Build history of the part. All positions in model axes, mm. Give positions to 0.01 mm unless a question says otherwise; leave off trailing zeros. Loops run counter-clockwise (first coordinate to the right, second up) from the corner with the lowest first, then second, coordinate; pieces in that order, holes last. Notation, with made-up numbers: (74.5, 0.25) -> (111.5, 0.25) arc R27 cw to (111.5, 35.25) -> close; hole circle Ø3 at (-29, 56.25). An arc over 180 degrees is marked (long way). Answer in a Markdown table with one row per item. Add a question column.
from build123d import *

# Parameters (mm, degrees)
ESQUISSE1_R                  = 3.5
ESQUISSE1_R_2                = 3
BOSS_EXTRU_1_DEPTH           = 314
ESQUISSE2_R                  = 1
ENL_V_MAT_EXTRU_1_DEPTH      = 10
ENL_V_MAT_EXTRU_1_DEPTH_BACK = 10


with BuildPart() as part:
    # Esquisse1 → Boss.-Extru.1 (new body)
    with BuildSketch(Plane.XY):
        Circle(ESQUISSE1_R)
        Circle(ESQUISSE1_R_2, mode=Mode.SUBTRACT)
    extrude(amount=BOSS_EXTRU_1_DEPTH)

    # Esquisse2 → Enl_v. mat.-Extru.1 (cut, two sides)
    with BuildSketch(Plane(origin=(0, 0, 0), x_dir=(1, 0, 0), z_dir=(0, 1, 0))) as enl_v_mat_extru_1_sk:
        with Locations((0, -309)):
            Circle(ESQUISSE2_R)
        with Locations((0, -5)):
            Circle(ESQUISSE2_R)
    extrude(amount=ENL_V_MAT_EXTRU_1_DEPTH, mode=Mode.SUBTRACT)
    extrude(enl_v_mat_extru_1_sk.sketch, amount=-ENL_V_MAT_EXTRU_1_DEPTH_BACK, mode=Mode.SUBTRACT)


solid = part.part
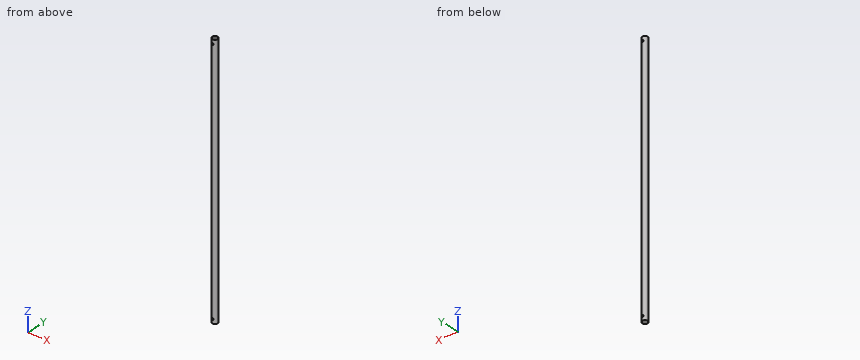
(1) Wall check: line 1 along Z through (x, y) = (0, 3.3); line 2 along Y through (x, z) = (-0.25, 168). Give the ranges that are in metal, low to high. Write a range as from..to.
(2) Flat gauge pins, fed straight in: pin 1 Ø3 at (y, z) = (1, 142) entering from +X; pin 2 Ø1.2 at (x, z) = (0, 309) entering from -Y. Where does each tip first touch, or does it go through?
(3) Saw through at A-A, the plane y = 0. List the corners of the cut face in (x, z).
(4) Saw through at B-B, the plane z = 230.5. List the corners of the cut face in (x, y).
Worked answers:
| question | item | result |
|---|---|---|
| 1 | line 1 | 0..4, 6..308, 310..314 |
| 1 | line 2 | -3.49..-2.99, 2.99..3.49 |
| 2 | pin 1 | x = 3.5 |
| 2 | pin 2 | through |
| 3 | outline | (-3.5, 0) -> (-3, 0) -> (-3, 314) -> (-3.5, 314) -> close; (3, 0) -> (3.5, 0) -> (3.5, 314) -> (3, 314) -> close |
| 4 | outline | circle Ø7 at (0, 0); hole circle Ø6 at (0, 0) |
